The model under review builds one solid part; all positions refer to its coordinate system, in mm. A direction names the side the tool comes from. Coordinates: 2 decimals unless noted, no trailing zeros. Order: outer loops, then holes, each group sorted by start corner. A loop starts at its lowest first (then second) coordinate and runs counter-clockwise, first axis right, second up. Notation, with made-up numbers: M -28,29 L 5,29 A27 ccw 5,48 Z; hole C 81,-20 d4. An arc over 180 degrees is marked long. Answer in a Markdown table with one row per item.
from build123d import *

# Parameters (mm, degrees)
SKETCH1_R           = 50
BOSS_EXTRUDE1_DEPTH = 400
SHELL1_T            = -10
SKETCH2_R           = 40
CUT_EXTRUDE1_DEPTH  = 400
SKETCH3_W           = 70
SKETCH3_H           = 40
CUT_EXTRUDE2_DEPTH  = 200
SKETCH4_R           = 45
CUT_EXTRUDE3_DEPTH  = 400
CUT_EXTRUDE7_DEPTH  = 75
BOSS_EXTRUDE3_START = -325
SKETCH9_W           = 40
SKETCH9_H           = 5.514468209
BOSS_EXTRUDE3_DEPTH = 365
SKETCH10_R          = 7.5
CUT_EXTRUDE8_DEPTH  = 454.081202098


with BuildPart() as part:
    # Sketch1 → Boss-Extrude1 (new body)
    with BuildSketch(Plane(origin=(0, 0, 0), x_dir=(1, 0, 0), z_dir=(0, 1, 0))):
        with Locations(Location((0, 0, 0), (0, 0, 90))):
            Circle(SKETCH1_R)
    extrude(amount=BOSS_EXTRUDE1_DEPTH)

    # Shell1
    shell1_openings = [part.faces().sort_by_distance(p)[0] for p in [
        (0, 0, 0),
    ]]
    offset(amount=SHELL1_T, openings=shell1_openings, kind=Kind.INTERSECTION)

    # Sketch2 → Cut-Extrude1 (cut)
    with BuildSketch(Plane.XZ.offset(-390)):
        with Locations(Location((0, 0, 0), (0, 0, 270))):
            Circle(SKETCH2_R)
    extrude(amount=-CUT_EXTRUDE1_DEPTH, mode=Mode.SUBTRACT)

    # Sketch3 → Cut-Extrude2 (cut, symmetric)
    with BuildSketch(Plane.XY):
        with Locations((0, 355)):
            Rectangle(SKETCH3_W, SKETCH3_H)
        with Locations((0, 280)):
            Rectangle(SKETCH3_W, SKETCH3_H)
        with Locations((0, 205)):
            Rectangle(SKETCH3_W, SKETCH3_H)
        with Locations((0, 130)):
            Rectangle(SKETCH3_W, SKETCH3_H)
        with Locations((0, 55)):
            Rectangle(SKETCH3_W, SKETCH3_H)
    extrude(amount=CUT_EXTRUDE2_DEPTH, both=True, mode=Mode.SUBTRACT)

    # Sketch4 → Cut-Extrude3 (cut)
    with BuildSketch(Plane(origin=(0, 400, 0), x_dir=(1, 0, 0), z_dir=(0, 1, 0))):
        with Locations(Location((0, 0, 0), (0, 0, 270))):
            Circle(SKETCH4_R)
    extrude(amount=-CUT_EXTRUDE3_DEPTH, mode=Mode.SUBTRACT)

    # Sketch8 → Cut-Extrude7 (cut)
    with BuildSketch(Plane(origin=(0, 0, 0), x_dir=(1, 0, 0), z_dir=(0, 1, 0))):
        Polygon((-283.60679775, 0), (-50, 0), (50, 0), (283.60679775, 0), (283.60679775, 467.2135955), (-283.60679775, 467.2135955), align=None)
    extrude(amount=CUT_EXTRUDE7_DEPTH, mode=Mode.SUBTRACT)

    # Sketch9 → Boss-Extrude3 (add)
    with BuildSketch(Plane(origin=(0, 400, 0), x_dir=(1, 0, 0), z_dir=(0, 1, 0)).offset(BOSS_EXTRUDE3_START)):
        with Locations((0, 43.068522846)):
            Rectangle(SKETCH9_W, SKETCH9_H)
        with Locations((0, -43.068522846)):
            Rectangle(SKETCH9_W, SKETCH9_H)
    extrude(amount=BOSS_EXTRUDE3_DEPTH)

    # Sketch10 → Cut-Extrude8 (cut, through all)
    with BuildSketch(Plane(origin=(0, 0, -45.82575695), x_dir=(-1, 0, 0), z_dir=(0, 0, -1))):
        with Locations((0, 420)):
            Circle(SKETCH10_R)
    extrude(amount=-CUT_EXTRUDE8_DEPTH, mode=Mode.SUBTRACT)


solid = part.part
(1) To check wall thickness, follow line 1 (Y direction, x = 0, z = -41.55); line 2 (X direction, y = 420, z = -43.7); line 3 (X direction, y = 255, z = 0). State the ranges of each line that lie inside material, in increasing order. Write a range as [from, to].
Report:
| item | result |
|---|---|
| line 1 | [75, 412.5], [427.5, 440] |
| line 2 | [-20, -7.5], [7.5, 20] |
| line 3 | [-50, -45], [45, 50] |
(2) Insertion check: P1, Ø3, axis at y = 138.5, z = 42, coming from the -X side; P2, Ø5, axis at y = 161.5, z = -35.5, coming from the +X side; P3, Ø8, axis at y = 130, z = -22.5, coming from the -X side. Each pin has a flat end and moves straight along its axis. Give the tip position at first contact, or say it passes through.
Report:
| item | result |
|---|---|
| P1 | x = -20 |
| P2 | x = 37.56 |
| P3 | x = -46.45 |
(3) The part is to be moulded in two halves that separate along Y. For faces 3 (the flat face through (-0.2, 0, 45.5)), 4 (the flat face through (-28, 375, 38)), 5 (the flat face through (45, 400, 4)), say which applies: +Y half, -Y half, draft (parallel to the pull), parting line (faces both ways), or undercut.
Report:
| item | result |
|---|---|
| face 3 | -Y half |
| face 4 | undercut |
| face 5 | +Y half |
(4) Take a section at D-D (y = 420). Write out the cut boundary in (x, z), then the cut area to 3 significant figures.
Report:
| item | result |
|---|---|
| outline | M -20,-45.83 L -7.5,-45.83 L -7.5,-40.31 L -20,-40.31 Z; M -20,40.31 L -7.5,40.31 L -7.5,45.83 L -20,45.83 Z; M 7.5,-45.83 L 20,-45.83 L 20,-40.31 L 7.5,-40.31 Z; M 7.5,40.31 L 20,40.31 L 20,45.83 L 7.5,45.83 Z |
| area | 276 mm^2 |
(5) Machinability: for faces 1 (the flat face through (-28, 335, 38)), 2 (the flat face through (0, 130, 45.826)), which of the approach directions +Z, -Z, +X, -X, +Y, -Y give a long, thin tool a straight path to every point of the face, cutting with its end or side? Answer none if there is none.
Report:
| item | result |
|---|---|
| face 1 | +Z, -Z |
| face 2 | +Z, +X, -X |
(6) Take a section at A-A (y = 132.5). Write out the cut boundary in (x, z), then the cut area to 3 significant figures.
Report:
| item | result |
|---|---|
| outline | M -35,-35.71 L -35,-28.28 A45 cw -35,28.28 L -35,35.71 A50 ccw Z; M -20,-45.83 L 20,-45.83 L 20,-40.31 L -20,-40.31 Z; M -20,40.31 L 20,40.31 L 20,45.83 L -20,45.83 Z; M 35,-35.71 A50 ccw 35,35.71 L 35,28.28 A45 cw 35,-28.28 Z |
| area | 1,150 mm^2 |
(7) Take a section at C-C (x = 0). State how many separate pieces and enclosed holes the cut face has, then the cut area to 3 significant figures.
Report:
| item | result |
|---|---|
| separate pieces | 5 |
| enclosed holes | 0 |
| area | 5,410 mm^2 |
(8) Take a section at B-B (z = -19). Write out the cut boundary in (x, y), then the cut area to 3 significant figures.
Report:
| item | result |
|---|---|
| outline | M -46.25,75 L -40.79,75 L -40.79,400 L -46.25,400 Z; M 40.79,75 L 46.25,75 L 46.25,400 L 40.79,400 Z |
| area | 3,550 mm^2 |
